Geometry check sheet. Reference: the model listing, model coordinates, mm. A direction names the side the tool comes from. Coordinates: 2 decimals unless noted, no trailing zeros. Loops run counter-clockwise (first coordinate to the right, second up) from the corner with the lowest first, then second, coordinate; pieces in that order, holes last. Notation, with made-up numbers: (-3, 22) - (20, 22) arc R30 cw to (20, 56) - close; hole circle Ø7 at (-15.75, 30). An arc over 180 degrees is marked (long way). Write each question's results on one line, items separated by ' | '. Start each with the question number.
(1) Mould release check, pull along Z, two halves, no side actions. Record for faces 3 (the face through (100.979, 3.042, -61.445)), 4 (the face through (-7.85, 2.96, -46.99)), 5 (the face through (-110, 3, 1)): pulls with the +Z half, pulls with the -Z half, needs draft (parallel to the pull), parting line crosses it, or undercut.
(2) Sectioned sample at C-C (y = 2.75). State how many separate pieces and enclosed holes the cut face has, plus the area to 3 significant figures.
(3) Material ranges on probe 1 along Z at (x, y) = (-74, 0.85); probe 2 along X at (y, z) = (4.65, -15.5); probe 3 along X at (y, z) = (5.25, -8.5), recorded low to high.
(4) Sectioned sample at A-A (x = -35). Enter the section's corners in (y, z), plus the area to 3 significant figures.
(5) Go/stop test with flat-tipped pins: pin 1 Ø2 at (x, z) = (-3.5, 22) entering from -Y; pin 2 Ø2 at (y, z) = (4, 46) entering from +X. Record where each tip stops, or that it passes through.
(6) Sectioned sample at B-B (z = 36). Enter the section's corners in (x, y).
(7) Access from +Z, -Z, +X, -X, +Y, -Y to the whole of each face (thin tool, end or side, straight path). Record for faces 1 (the face through (-7.85, 2.96, 8.01)), 2 (the face through (100.979, 3.042, 61.445)).
from build123d import *

# Parameters (mm, degrees)
ESBO_O1_W                = 220
ESBO_O1_H                = 140
RESSALTO_EXTRUS_O1_DEPTH = 6
ESBO_O2_W                = 85
ESBO_O2_H                = 45
CORTE_EXTRUS_O1_DEPTH    = 6
FILETE1_R                = 30
FILETE2_R                = 10


with BuildPart() as part:
    # Esboço1 → Ressalto-extrusão1 (new body)
    with BuildSketch(Plane(origin=(0, 0, 0), x_dir=(1, 0, 0), z_dir=(0, 1, 0))):
        Rectangle(ESBO_O1_W, ESBO_O1_H)
    extrude(amount=RESSALTO_EXTRUS_O1_DEPTH)

    # Esboço2 → Corte-extrusão1 (cut)
    with BuildSketch(Plane(origin=(0, 6, 0), x_dir=(1, 0, 0), z_dir=(0, 1, 0))):
        with Locations((47.5, 27.5)):
            Rectangle(ESBO_O2_W, ESBO_O2_H)
        with Locations((-47.5, 27.5)):
            Rectangle(ESBO_O2_W, ESBO_O2_H)
        with Locations((-47.5, -27.5)):
            Rectangle(ESBO_O2_W, ESBO_O2_H)
        with Locations((47.5, -27.5)):
            Rectangle(ESBO_O2_W, ESBO_O2_H)
    extrude(amount=-CORTE_EXTRUS_O1_DEPTH, mode=Mode.SUBTRACT)

    # Filete1
    filete1_edges = [part.edges().sort_by_distance(p)[0] for p in [
        (-110, 3, -70),
        (110, 3, -70),
        (110, 3, 70),
        (-110, 3, 70),
    ]]
    fillet(filete1_edges, radius=FILETE1_R)

    # Filete2
    filete2_edges = [part.edges().sort_by_distance(p)[0] for p in [
        (-90, 3, -50),
        (-5, 3, -50),
        (-5, 3, -5),
        (-90, 3, -5),
        (-90, 3, 50),
        (-90, 3, 5),
        (-5, 3, 5),
        (-5, 3, 50),
        (90, 3, 50),
        (5, 3, 50),
        (5, 3, 5),
        (90, 3, 5),
        (5, 3, -50),
        (90, 3, -50),
        (90, 3, -5),
        (5, 3, -5),
    ]]
    fillet(filete2_edges, radius=FILETE2_R)


solid = part.part
Outcome:
1) face 3: pulls with the -Z half | face 4: undercut | face 5: needs draft
2) separate pieces: 1 | enclosed holes: 4 | area: 15,100 mm2
3) probe 1: z = -70 to -50, -5 to 5, 50 to 70 | probe 2: x = -110 to -90, -5 to 5, 90 to 110 | probe 3: x = -110 to -87.6, -7.4 to 7.4, 87.6 to 110
4) outline: (0, -70) - (6, -70) - (6, -50) - (0, -50) - close; (0, -5) - (6, -5) - (6, 5) - (0, 5) - close; (0, 50) - (6, 50) - (6, 70) - (0, 70) - close | area: 300 mm2
5) pin 1: stops at y = 0 | pin 2: stops at x = 109.58
6) outline: (-110, 0) - (-90, 0) - (-90, 6) - (-110, 6) - close; (-5, 0) - (5, 0) - (5, 6) - (-5, 6) - close; (90, 0) - (110, 0) - (110, 6) - (90, 6) - close
7) face 1: +Y, -Y | face 2: +Z, +X, +Y, -Y
